```python
from build123d import *

# Parameters (mm, degrees)
SKETCH1_W           = 9.848024316
SKETCH1_H           = 16
BOSS_EXTRUDE1_DEPTH = 9
SKETCH3_R           = 3.05
CUT_EXTRUDE1_DEPTH  = 9
SKETCH4_W           = 8.110790477
SKETCH4_H           = 20.153934792
CUT_EXTRUDE2_DEPTH  = 9


with BuildPart() as part:
    # Sketch1 → Boss-Extrude1 (new body)
    with BuildSketch(Plane(origin=(0, 0, 0), x_dir=(0, 0, -1), z_dir=(1, 0, 0))):
        Rectangle(SKETCH1_W, SKETCH1_H)
    extrude(amount=BOSS_EXTRUDE1_DEPTH)

    # Sketch3 → Cut-Extrude1 (cut)
    with BuildSketch(Plane.ZY):
        with Locations((0, 3.5)):
            Circle(SKETCH3_R)
        with Locations((0, -4)):
            Circle(SKETCH3_R)
    extrude(amount=-CUT_EXTRUDE1_DEPTH, mode=Mode.SUBTRACT)

    # Sketch4 → Cut-Extrude2 (cut)
    with BuildSketch(Plane.ZY):
        with Locations((4.055395239, 0)):
            Rectangle(SKETCH4_W, SKETCH4_H)
    extrude(amount=-CUT_EXTRUDE2_DEPTH, mode=Mode.SUBTRACT)


solid = part.part
```
Build history of the part. All positions in model axes, mm. Give positions to 0.01 mm unless a question says otherwise; leave off trailing zeros. Loops run counter-clockwise (first coordinate to the right, second up) from the corner with the lowest first, then second, coordinate; pieces in that order, holes last.
Item 1: Slice it at D-D, the plane y = 3.5. List the corners of the cut face in (x, z), and give its area (3 significant figures).
Answers follow:
outline: (0, -4.92) - (9, -4.92) - (9, -3.05) - (0, -3.05) - close
area: 16.9 mm2
Item 2: Pull direction Y, two halves, no side cores. Call faces 1 (the face through (9, 0, -3)), 2 (the face through (4, 8, -2)), 3 (the face through (4.44, 3.57, -3.05)): released by +Y, released by -Y, zero draft, split by the parting line, or undercut.
Answers follow:
face 1: zero draft
face 2: released by +Y
face 3: undercut
Item 3: Drill centre lines: line 1 (Y direction, x = 8.5, z = -1); line 2 (Y direction, x = 3.5, z = -0.6); line 3 (Z direction, x = 2.25, y = 3.75). Where is each one in solid material? Low to high.
Answers follow:
line 1: y = -8 to -6.88, -1.12 to 0.62, 6.38 to 8
line 2: y = -8 to -6.99, -1.01 to 0.51, 6.49 to 8
line 3: z = -4.92 to -3.04
Item 4: Flat gauge pin, fed straight in: pin 1 (1 mm diameter, centred on x = 3.5, y = 3.5, fed in from +Z). Where does the tip first touch, or does it go through?
Answers follow:
pin 1: stops at z = -3.01
Item 5: Slice it at C-C, the plane z = -2.75. List the corners of the cut face in (x, y).
Answers follow:
outline: (0, -8) - (9, -8) - (9, -5.32) - (0, -5.32) - close; (0, -2.68) - (9, -2.68) - (9, 2.18) - (0, 2.18) - close; (0, 4.82) - (9, 4.82) - (9, 8) - (0, 8) - close
Item 6: Slice it at B-B, the plane x = 2.25. List the corners of the cut face in (y, z).
Answers follow:
outline: (-8, -4.92) - (8, -4.92) - (8, 0) - (6.55, 0) arc R3.05 cw to (0.45, 0) - (-0.95, 0) arc R3.05 cw to (-7.05, 0) - (-8, 0) - close
Item 7: Slice it at A-A, the plane z = -0.45. List the corners of the cut face in (x, y), and give its area (3 significant figures).
Answers follow:
outline: (0, -8) - (9, -8) - (9, -7.02) - (0, -7.02) - close; (0, -0.98) - (9, -0.98) - (9, 0.48) - (0, 0.48) - close; (0, 6.52) - (9, 6.52) - (9, 8) - (0, 8) - close
area: 35.4 mm2
